Here's how the part is built. I have some questions about the finished solid (model axes, mm). Face numbers are marked on the shaded views. A direction names the side the tool comes from. Round coordinates to 2 decimals unless told otherwise and drop trailing zeros. Order: outer loops, then holes, each group sorted by start corner. A loop starts at its lowest first (then second) coordinate and runs counter-clockwise, first axis right, second up. Notation, with made-up numbers: (1, 85.5) -> (11, 85.5) arc R29 cw to (11, 115.5) -> close; hole circle Ø3 at (-31.75, -19). An arc over 180 degrees is marked (long way). One line per item, written item: value.
```python
from build123d import *

# Parameters (mm, degrees)
SKETCH_1_W      = 70
SKETCH_1_H      = 50
EXTRUDE_1_DEPTH = 2
FILLET_1_R      = 3
SKETCH_2_W      = 2
SKETCH_2_H      = 44
EXTRUDE_2_DEPTH = 5
SKETCH_3_R      = 0.91
EXTRUDE_3_DEPTH = 2.5


with BuildPart() as part:
    # 草图1 → 凸台-拉伸1 (new body)
    with BuildSketch(Plane(origin=(0, 0, 0), x_dir=(1, 0, 0), z_dir=(0, 1, 0))):
        Rectangle(SKETCH_1_W, SKETCH_1_H)
    extrude(amount=EXTRUDE_1_DEPTH)

    # 圆角1
    fillet_1_edges = [part.edges().sort_by_distance(p)[0] for p in [
        (35, 1, 25),
        (-35, 1, 25),
        (-35, 1, -25),
        (35, 1, -25),
    ]]
    fillet(fillet_1_edges, radius=FILLET_1_R)

    # 草图2 → 凸台-拉伸2 (add)
    with BuildSketch(Plane(origin=(0, 2, 0), x_dir=(1, 0, 0), z_dir=(0, 1, 0))):
        with Locations((-34, 0)):
            Rectangle(SKETCH_2_W, SKETCH_2_H)
        with Locations((34, 0)):
            Rectangle(SKETCH_2_W, SKETCH_2_H)
    extrude(amount=EXTRUDE_2_DEPTH)

    # 草图3 → 凸台-拉伸3 (add)
    # profile 1 of 2: a face of its own
    with BuildSketch(Plane(origin=(0, 2, 0), x_dir=(1, 0, 0), z_dir=(0, 1, 0))):
        with BuildLine():
            Line((28, 22.985971126), (19, 22.985971126))
            Line((19, 22.985971126), (19, 15.46603773))
            Line((19, 15.46603773), (27.222114772, 7.243922958))
            Line((27.222114772, 7.243922958), (27.222114772, -11.014028874))
            Line((27.222114772, -11.014028874), (31, -11.014028874))
            Line((31, -11.014028874), (31, 19.985971126))
            ThreePointArc((31, 19.985971126), (30.121320344, 22.10729147), (28, 22.985971126))
        make_face()
        with Locations(Location((24, 20.49257992, 0), (0, 0, 270))):
            Circle(SKETCH_3_R, mode=Mode.SUBTRACT)
    # profile 2 of 2: a face of its own
    with BuildSketch(Plane(origin=(0, 2, 0), x_dir=(1, 0, 0), z_dir=(0, 1, 0))):
        with BuildLine():
            Line((-28, 22), (-26, 22))
            Line((-26, 22), (-26, -16.071759555))
            Line((-26, -16.071759555), (-28, -16.071759555))
            ThreePointArc((-28, -16.071759555), (-30.121320344, -15.193079899), (-31, -13.071759555))
            Line((-31, -13.071759555), (-31, 19))
            ThreePointArc((-31, 19), (-30.121320344, 21.121320344), (-28, 22))
        make_face()
    extrude(amount=EXTRUDE_3_DEPTH)


solid = part.part
```
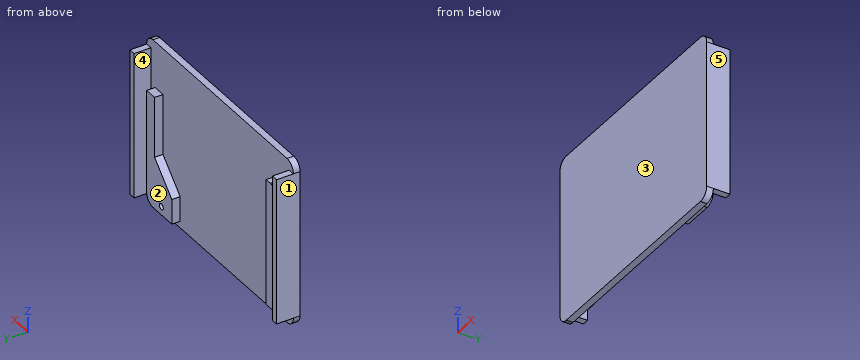
Q1. I want a section at C-C on x = 20.5. Write out the boundary of the cut face in (y, z), then the cut area to 3 significant figures.
Answers:
outline: (0, -25) -> (2, -25) -> (2, -22.99) -> (4.5, -22.99) -> (4.5, -13.97) -> (2, -13.97) -> (2, 25) -> (0, 25) -> close
area: 123 mm2
Q2. For P1, Ø2, axis at x = 34.5, y = 4.5, coming from the +Z side; P2, Ø1.6, axis at x = 24, z = -20.49, coming from the +Y side; P3, Ø2, axis at x = -27, y = 3.5, coming from the -Z side, each with a flat end and sliding along its axis, tell me the tip position at first contact or that it passes through.
Answers:
P1: z = 22
P2: y = 2
P3: z = -22
Q3. I want a section at D-D on z = -2.5. Write out the boundary of the cut face in (x, y), then the cut area to 3 significant figures.
Answers:
outline: (-35, 0) -> (35, 0) -> (35, 7) -> (33, 7) -> (33, 2) -> (31, 2) -> (31, 4.5) -> (27.22, 4.5) -> (27.22, 2) -> (-26, 2) -> (-26, 4.5) -> (-31, 4.5) -> (-31, 2) -> (-33, 2) -> (-33, 7) -> (-35, 7) -> close
area: 182 mm2
Q4. If we mould it in two halves opening along X, with no side actions, what happens to the marked faces 1, 2 and 3? For each: pulls with the +X half, pulls with the -X half, needs draft (parallel to the pull), parting line crosses it, or undercut.
Answers:
face 1: pulls with the -X half
face 2: undercut
face 3: needs draft
Q5. I need wall thicknesses on line 1 along X through (y, z) = (3.75, 6); line 2 along X through (y, z) = (5.5, -8.5); line 3 along X through (y, z) = (2.75, -10.5). Which ranges of each line are inside material? Lowest first, please.
Answers:
line 1: -35 to -33, -31 to -26, 27.22 to 31, 33 to 35
line 2: -35 to -33, 33 to 35
line 3: -35 to -33, -31 to -26, 23.97 to 31, 33 to 35
Q6. I want a section at A-A on y = 3.5. Write out the boundary of the cut face in (x, z).
Answers:
outline: (-35, -22) -> (-33, -22) -> (-33, 22) -> (-35, 22) -> close; (-31, -19) arc R3 ccw to (-28, -22) -> (-26, -22) -> (-26, 16.07) -> (-28, 16.07) arc R3 ccw to (-31, 13.07) -> close; (19, -22.99) -> (28, -22.99) arc R3 ccw to (31, -19.99) -> (31, 11.01) -> (27.22, 11.01) -> (27.22, -7.24) -> (19, -15.47) -> close; (33, -22) -> (35, -22) -> (35, 22) -> (33, 22) -> close; hole circle Ø1.82 at (24, -20.49)
Q7. Which directions (+Z, -Z, +X, -X, +Y, -Y) give clear straight access to the entire face, cutting with the end or side of a thin tool? Please do the marked faces 4 and 5.
Answers:
face 4: +Z, -Z, +Y
face 5: +Z, -Z, +X, +Y, -Y
Q8. I want a section at B-B on z = -17.5. Write out the boundary of the cut face in (x, y), then the cut area to 4 significant figures.
Answers:
outline: (-35, 0) -> (35, 0) -> (35, 7) -> (33, 7) -> (33, 2) -> (31, 2) -> (31, 4.5) -> (19, 4.5) -> (19, 2) -> (-26, 2) -> (-26, 4.5) -> (-31, 4.5) -> (-31, 2) -> (-33, 2) -> (-33, 7) -> (-35, 7) -> close
area: 202.5 mm2
